from build123d import *

# Parameters (mm, degrees)
SKETCH1_W           = 119
SKETCH1_H           = 6
BOSS_EXTRUDE1_DEPTH = 4
CUT_EXTRUDE1_REACH  = 6
SKETCH2_W           = 3
SKETCH2_H           = 3
SKETCH3_W           = 10
SKETCH3_H           = 4
BOSS_EXTRUDE2_DEPTH = 26
SKETCH4_W           = 10
SKETCH4_H           = 6
BOSS_EXTRUDE3_DEPTH = 20
SKETCH5_W           = 6
SKETCH5_H           = 4
BOSS_EXTRUDE4_DEPTH = 42.5


with BuildPart() as part:
    # Sketch1 → Boss-Extrude1 (new body)
    with BuildSketch(Plane(origin=(0, 0, 0), x_dir=(1, 0, 0), z_dir=(0, 1, 0))):
        with Locations((59.5, 3)):
            Rectangle(SKETCH1_W, SKETCH1_H)
    extrude(amount=BOSS_EXTRUDE1_DEPTH)

    # Sketch2 → Cut-Extrude1 (cut, up to next)
    with BuildSketch(Plane(origin=(0, 4, 0), x_dir=(1, 0, 0), z_dir=(0, 1, 0)), mode=Mode.PRIVATE) as cut_extrude1_sk1:
        with Locations((114.5, 3)):
            Rectangle(SKETCH2_W, SKETCH2_H)
    cut_extrude1_tool1 = extrude(cut_extrude1_sk1.sketch, amount=-CUT_EXTRUDE1_REACH, mode=Mode.PRIVATE) & part.part
    add(cut_extrude1_tool1.solids().sort_by_distance((114.5, 4, -3))[0], mode=Mode.SUBTRACT)
    # Sketch2 → Cut-Extrude1 (cut, up to next)
    with BuildSketch(Plane(origin=(0, 4, 0), x_dir=(1, 0, 0), z_dir=(0, 1, 0)), mode=Mode.PRIVATE) as cut_extrude1_sk2:
        with Locations((4.5, 3)):
            Rectangle(SKETCH2_W, SKETCH2_H)
    cut_extrude1_tool2 = extrude(cut_extrude1_sk2.sketch, amount=-CUT_EXTRUDE1_REACH, mode=Mode.PRIVATE) & part.part
    add(cut_extrude1_tool2.solids().sort_by_distance((4.5, 4, -3))[0], mode=Mode.SUBTRACT)

    # Sketch3 → Boss-Extrude2 (add)
    with BuildSketch(Plane(origin=(0, 0, -6), x_dir=(-1, 0, 0), z_dir=(0, 0, -1))):
        with Locations((-105, 2)):
            Rectangle(SKETCH3_W, SKETCH3_H)
        with Locations((-81.5, 2)):
            Rectangle(SKETCH3_W, SKETCH3_H)
        with Locations((-14, 2)):
            Rectangle(SKETCH3_W, SKETCH3_H)
    extrude(amount=BOSS_EXTRUDE2_DEPTH)

    # Sketch4 → Boss-Extrude3 (add)
    with BuildSketch(Plane.XZ):
        with Locations((105, -3)):
            Rectangle(SKETCH4_W, SKETCH4_H)
        with Locations((81.5, -3)):
            Rectangle(SKETCH4_W, SKETCH4_H)
        with Locations((14, -3)):
            Rectangle(SKETCH4_W, SKETCH4_H)
    extrude(amount=BOSS_EXTRUDE3_DEPTH)

    # Sketch5 → Boss-Extrude4 (add)
    with BuildSketch(Plane.ZY.offset(-76.5)):
        with Locations((-25, 2)):
            Rectangle(SKETCH5_W, SKETCH5_H)
        with Locations((-3, -18)):
            Rectangle(SKETCH5_W, SKETCH5_H)
    extrude(amount=-BOSS_EXTRUDE4_DEPTH)


solid = part.part
Verification items for the finished model (mm, model axes). A direction names the side the tool comes from. Round coordinates to 2 decimals unless told otherwise and drop trailing zeros. Loops run counter-clockwise (first coordinate to the right, second up) from the corner with the lowest first, then second, coordinate; pieces in that order, holes last. Notation, with made-up numbers: (2, 21) - (42, 21) arc R34 cw to (42, 60) - close; hole circle Ø6 at (34, 82). An arc over 180 degrees is marked (long way). Answer in a Markdown table with one row per item. Add a question column.
Q1. Material ranges on line 1 (X direction, y = 1.75, z = -29); line 2 (X direction, y = 3, z = -25); line 3 (Y direction, x = 11, z = -28), recorded low to high.
Q2. Section check A-A on z = -10. Enter the section's corners in (x, y), plus the area to 3 significant figures.
Q3. Section check B-B on y = -1.5. Enter the section's corners in (x, z).
Q4. Release check for a two-part mould opening along Z. For faces 4 (the face through (4, 2, -6)), 5 (the face through (3, 2, -3)), 6 (the face through (97, 0, -25)) record: pulls with the +Z half, pulls with the -Z half, needs draft (parallel to the pull), parting line crosses it, or undercut.
Q5. Section check D-D on x = 13. Enter the section's corners in (y, z).
Q6. Section check C-C on z = -24.5. Enter the section's corners in (x, y).
Q7. Gauge pin test, flat ends, axial feed: pin 1 (4.5 mm diameter, centred on x = 113.5, y = 3, fed in from -Z); pin 2 (8 mm diameter, centred on y = 1, z = -16, fed in from +X); pin 3 (8 mm diameter, centred on x = 87.5, y = -9, fed in from -Z). Record the tip position at first contact, or that the pin passes through.
Q8. Tool access check on faces 1 (the face through (9, -10, -3)), 2 (the face through (47, 2, -6)), 3 (the face through (4, 2, -4.5)). Record the directions out of +Z, -Z, +X, -X, +Y, -Y that give a thin tool (end or side, any length) a straight path to the whole face; none if there is none.
Found:
| question | item | result |
|---|---|---|
| 1 | line 1 | x = 9 to 19, 76.5 to 86.5, 100 to 110 |
| 1 | line 2 | x = 9 to 19, 76.5 to 119 |
| 1 | line 3 | y = 0 to 4 |
| 2 | outline | (9, 0) - (19, 0) - (19, 4) - (9, 4) - close; (76.5, 0) - (86.5, 0) - (86.5, 4) - (76.5, 4) - close; (100, 0) - (110, 0) - (110, 4) - (100, 4) - close |
| 2 | area | 120 mm² |
| 3 | outline | (9, -6) - (19, -6) - (19, 0) - (9, 0) - close; (76.5, -6) - (86.5, -6) - (86.5, 0) - (76.5, 0) - close; (100, -6) - (110, -6) - (110, 0) - (100, 0) - close |
| 4 | face 4 | pulls with the -Z half |
| 4 | face 5 | undercut |
| 4 | face 6 | needs draft |
| 5 | outline | (-20, -6) - (0, -6) - (0, -32) - (4, -32) - (4, 0) - (-20, 0) - close |
| 6 | outline | (9, 0) - (19, 0) - (19, 4) - (9, 4) - close; (76.5, 0) - (119, 0) - (119, 4) - (76.5, 4) - close |
| 7 | pin 1 | stops at z = -28 |
| 7 | pin 2 | stops at x = 110 |
| 7 | pin 3 | stops at z = -6 |
| 8 | face 1 | +Z, -Z, -X, -Y |
| 8 | face 2 | -Z, +Y, -Y |
| 8 | face 3 | +Y, -Y |
